Geometry: see drawing. Coordinates: mm, zero at the bounding-box minimum. A direction names the side the tool comes from. Give positions to 0.01 mm unless a question says otherwise; leave off trailing zeros. Order: outer loops, then holes, each group sorted by start corner. A loop starts at its lowest first (then second) coordinate and runs counter-clockwise, first axis right, second up. Notation, with made-up numbers: (24.5, -14.5) - (71.5, -14.5) arc R15 cw to (71.5, 13.5) - close; hole circle Ø2 at (1, -12.75). An arc over 180 degrees is marked (long way). Put each result on its own line as item: value. Start each with the question number.
1. Set-up query: the marked faces 1 and 2. Return all of +Z, -Z, +X, -X, +Y, -Y with unobstructed straight access to the full face (end or side cutting, diameter ignored); none if empty.
2. Section A-A on y = 7. Return the cut outline in (x, z), plus the area to 3 significant figures.
3. Section B-B on z = 5.45. Return the cut outline in (x, y), plus the area to 3 significant figures.
4. Section C-C on z = 1.6. Return the cut outline in (x, y), plus the area to 3 significant figures.
5. Ray query, line 1 along Z through (x, y) = (3.5, 6.75); line 2 along Z through (x, y) = (3.25, 12.5); line 3 along Y through (x, z) = (9, 1.6). Return the intervals inside material, ascending. Write a range as from..to.
6. Mould query, pull axis X, two halves, no side actions, for the marked faces 3 and 4. Classes: pulls with the +X half, pulls with the -X half, needs draft (parallel to the pull), parting line crosses it, or undercut.
7. First-contact query: P1, Ø3, axis at x = 10, z = 3, coming from the +Y side; P2, Ø4, axis at x = 8.5, y = 5, coming from the -Z side; P3, Ø1.5, axis at y = 4, z = 4.5, coming from the -X side; P4, Ø1, axis at y = 2, z = 0.5, coming from the -X side. Flat tips, straight axial feed; report the tip coordinate or a pass-through.
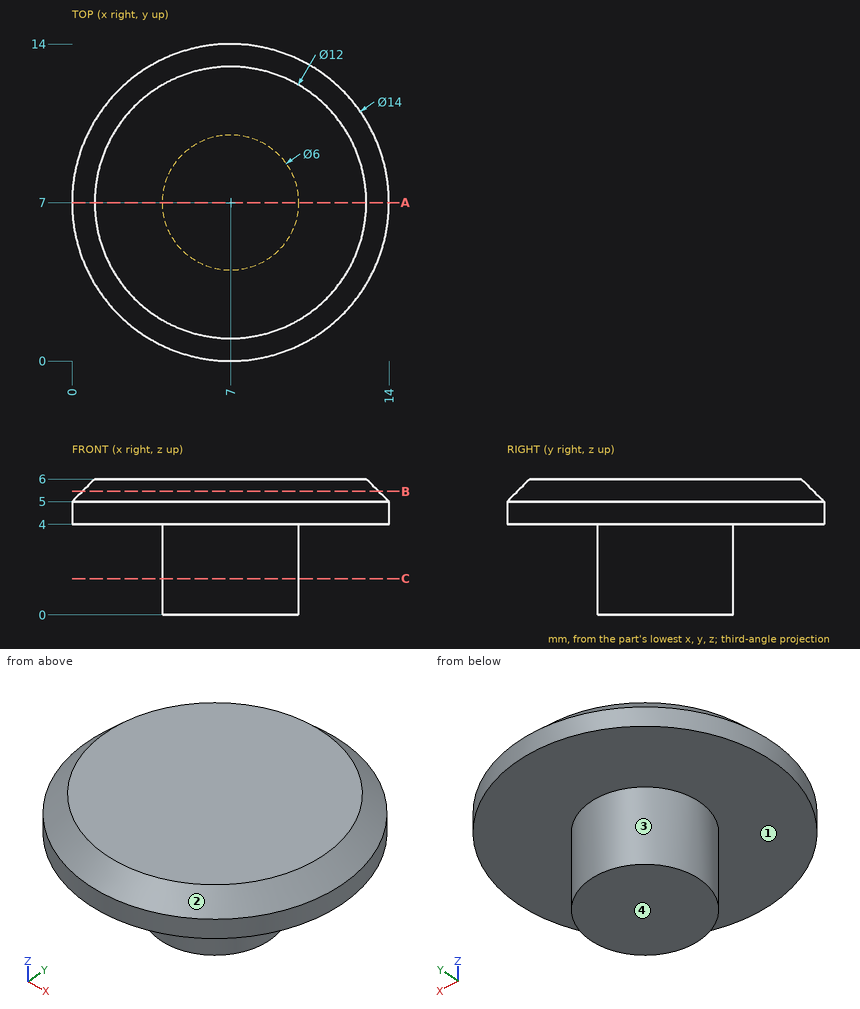
Resolved:
1. face 1: -Z
1. face 2: +Z
2. outline: (0, 4) - (4, 4) - (4, 0) - (10, 0) - (10, 4) - (14, 4) - (14, 5) - (13, 6) - (1, 6) - (0, 5) - close
2. area: 51.0 mm^2
3. outline: circle Ø13.1 at (7, 7)
3. area: 135 mm^2
4. outline: circle Ø6 at (7, 7)
4. area: 28.3 mm^2
5. line 1: 4..6
5. line 2: 4..5.34
5. line 3: 4.76..9.24
6. face 3: parting line crosses it
6. face 4: needs draft
7. P1: y = 13.74
7. P2: z = 0
7. P3: x = 0.37
7. P4: through
